Geometry: final body of the model. Coordinates: model frame, mm. A direction names the side the tool comes from. Coordinates: 2 decimals unless noted, no trailing zeros. Loops run counter-clockwise (first coordinate to the right, second up) from the corner with the lowest first, then second, coordinate; pieces in that order, holes last. Notation, with made-up numbers: (7.25, -9) - (42.25, -9) arc R12 ccw to (42.25, -1) - close; hole circle Ø1 at (-27, -5). An arc over 180 degrees is marked (long way). Return JSON: item names as keys, results as strings.
from build123d import *

# Parameters (mm, degrees)
F1_DEPTH = 30
F2_R     = 2.5
F3_DEPTH = 3
F4_R     = 6
F4_R_2   = 2.5
F5_DEPTH = 4
F6_R     = 2
F7_D     = 4
F7_DEPTH = 15
F7_TIP   = 1.2017212381


with BuildPart() as f1:
    # F0 (on Front) → F1 (new body)
    with BuildSketch(Plane.XZ):
        Polygon((0, 1), (0, 0), (18, 0), (18, 1), (18, 16), (17, 16), (17, 1), (1, 1), (1, 16), (0, 16), align=None)
    extrude(amount=-F1_DEPTH)

    # F2 (on face) → F3 (join)
    with BuildSketch(Plane.XY.offset(1)):
        with Locations((9, 15)):
            Circle(F2_R)
    extrude(amount=-F3_DEPTH)

    # F4 (on face) → F5 (join)
    with BuildSketch(Plane(origin=(0, 0, -2), x_dir=(1, 0, 0), z_dir=(0, 0, -1))):
        with Locations((9, -15)):
            Circle(F4_R)
        with Locations((9, -15)):
            Circle(F4_R_2, mode=Mode.SUBTRACT)
        with Locations((9, -15)):
            Circle(F4_R_2)
    extrude(amount=F5_DEPTH)

    # F6
    f6_edges = [f1.edges().sort_by_distance(p)[0] for p in [
        (17.5, 0, 16),
        (17.5, 30, 16),
        (0.5, 30, 16),
        (0.5, 0, 16),
    ]]
    fillet(f6_edges, radius=F6_R)

    # F7
    with Locations(Plane.XY.offset(1)):
        with Locations((9, 4), (9, 26)):
            Hole(F7_D / 2, depth=F7_DEPTH)
            with Locations((0, 0, -(F7_DEPTH + F7_TIP / 2))):  # 118° drill point
                Cone(0, F7_D / 2, F7_TIP, mode=Mode.SUBTRACT)


solid = f1.part
Item 1: Reachability of faces 1 (the face through (1, 15, 8)), 2 (the face through (9.434, 2.048, 0.493)) from +Z, -Z, +X, -X, +Y, -Y: full face, straight path, thin tool, end or side. Return the list, or none.
Worked out:
{"face 1": "+Z, +Y, -Y", "face 2": "+Z, -Z"}
Item 2: Section query D-D, the plane x = 14.5. Return loops of the section in (y, z).
Worked out:
{"outline": "(0, 0) - (30, 0) - (30, 1) - (0, 1) - close; (12.6, -6) - (17.4, -6) - (17.4, -2) - (12.6, -2) - close"}
Item 3: Section query B-B, the plane y = 27.5. Return loops of the section in (x, z).
Worked out:
{"outline": "(0, 0) - (7.68, 0) - (7.68, 1) - (1, 1) - (1, 16) - (0, 16) - close; (10.32, 0) - (18, 0) - (18, 16) - (17, 16) - (17, 1) - (10.32, 1) - close"}
Item 4: Mould query, pull axis Z, two halves, no side actions, for faces 3 (the face through (9, 18, -2)), 4 (the face through (9, 18, 0)), 5 (the face through (8.22, 9.05, -3.97)), 6 (the face through (9, 15, -6)). Classes: +Z half, -Z half, draft (parallel to the pull), parting line (faces both ways), or undercut.
Worked out:
{"face 3": "undercut", "face 4": "undercut", "face 5": "draft", "face 6": "-Z half"}
Item 5: Section query C-C, the plane y = 22.75. Return loops of the section in (x, z).
Worked out:
{"outline": "(0, 0) - (18, 0) - (18, 16) - (17, 16) - (17, 1) - (1, 1) - (1, 16) - (0, 16) - close"}
Item 6: First-contact query: pin 1 Ø5 at (x, y) = (9, 4) entering from -Z; pin 2 Ø1 at (x, z) = (9, 0.5) entering from -Y; pin 3 Ø5 at (x, y) = (12.5, 11) entering from +Z; pin 4 Ø3.5 at (x, y) = (9, 26) entering from +Z. Flat tips, straight axial feed; report the tip coordinate or a pass-through.
Worked out:
{"pin 1": "z = 0", "pin 2": "y = 0", "pin 3": "z = 1", "pin 4": "through"}
Item 7: Section query A-A, the plane x = 9. Return loops of the section in (y, z).
Worked out:
{"outline": "(0, 0) - (2, 0) - (2, 1) - (0, 1) - close; (6, 0) - (12.5, 0) - (12.5, -2) - (9, -2) - (9, -6) - (21, -6) - (21, -2) - (17.5, -2) - (17.5, 0) - (24, 0) - (24, 1) - (6, 1) - close; (28, 0) - (30, 0) - (30, 1) - (28, 1) - close"}
Item 8: Ray query, probe 1 along Y at (x, z) = (9, 0.55); probe 2 along Z at (x, y) = (4.5, 11.5); probe 3 along X at (y, z) = (13.5, 5.5). Return the intervals inside material, ascending. Write a range as from..to.
Worked out:
{"probe 1": "0..2, 6..24, 28..30", "probe 2": "-6..-2, 0..1", "probe 3": "0..1, 17..18"}
